```python
from build123d import *

# Parameters (mm, degrees)
SKETCH1_R           = 0.75
BOSS_EXTRUDE1_DEPTH = 2
SKETCH2_W           = 20.7
SKETCH2_H           = 2
SKETCH2_W_2         = 25.7
BOSS_EXTRUDE2_DEPTH = 4


with BuildPart() as part:
    # Sketch1 → Boss-Extrude1 (new body)
    # profile 1 of 3: a face of its own
    with BuildSketch(Plane(origin=(0, -22.368471217, 0), x_dir=(1, 0, 0), z_dir=(0, 1, 0))):
        Polygon((-7.325383597, 61.756641018), (1.674616403, 61.756641018), (1.674616403, 63.756641018), (-5.325383597, 63.756641018), (-5.325383597, 65.756641018), (-9.325383597, 65.756641018), (-9.325383597, 37.256641018), (-5.325383597, 37.256641018), (-5.325383597, 39.256641018), (1.674616403, 39.256641018), (1.674616403, 41.256641018), (-7.325383597, 41.256641018), align=None)
        with Locations(Location((-7.325383597, 63.756641018, 0), (0, 0, 270))):
            Circle(SKETCH1_R, mode=Mode.SUBTRACT)
        with Locations(Location((-7.325383597, 39.256641018, 0), (0, 0, 270))):
            Circle(SKETCH1_R, mode=Mode.SUBTRACT)
    # profile 2 of 3: a face of its own
    with BuildSketch(Plane(origin=(0, -22.368471217, 0), x_dir=(1, 0, 0), z_dir=(0, 1, 0))):
        Polygon((1.674616403, 39.256641018), (22.974616403, 39.256641018), (22.974616403, 41.256641018), (31.974616403, 41.256641018), (31.974616403, 61.756641018), (27.974616403, 61.756641018), (27.974616403, 63.756641018), (1.674616403, 63.756641018), (1.674616403, 61.756641018), (-7.325383597, 61.756641018), (-7.325383597, 41.256641018), (1.674616403, 41.256641018), align=None)
    # profile 3 of 3: a face of its own
    with BuildSketch(Plane(origin=(0, -22.368471217, 0), x_dir=(1, 0, 0), z_dir=(0, 1, 0))):
        Polygon((29.974616403, 65.756641018), (29.974616403, 63.756641018), (27.974616403, 63.756641018), (27.974616403, 61.756641018), (31.974616403, 61.756641018), (31.974616403, 41.256641018), (22.974616403, 41.256641018), (22.974616403, 39.256641018), (29.974616403, 39.256641018), (29.974616403, 37.256641018), (33.974616403, 37.256641018), (33.974616403, 65.756641018), align=None)
        with Locations(Location((31.974616403, 39.256641018, 0), (0, 0, 270))):
            Circle(SKETCH1_R, mode=Mode.SUBTRACT)
        with Locations(Location((31.974616403, 63.756641018, 0), (0, 0, 270))):
            Circle(SKETCH1_R, mode=Mode.SUBTRACT)
    extrude(amount=BOSS_EXTRUDE1_DEPTH)

    # Sketch2 → Boss-Extrude2 (add)
    with BuildSketch(Plane.XZ.offset(22.368471217)):
        with Locations((12.324616403, -40.256641018)):
            Rectangle(SKETCH2_W, SKETCH2_H)
        with Locations((14.824616403, -62.756641018)):
            Rectangle(SKETCH2_W_2, SKETCH2_H)
    extrude(amount=BOSS_EXTRUDE2_DEPTH)


solid = part.part
```
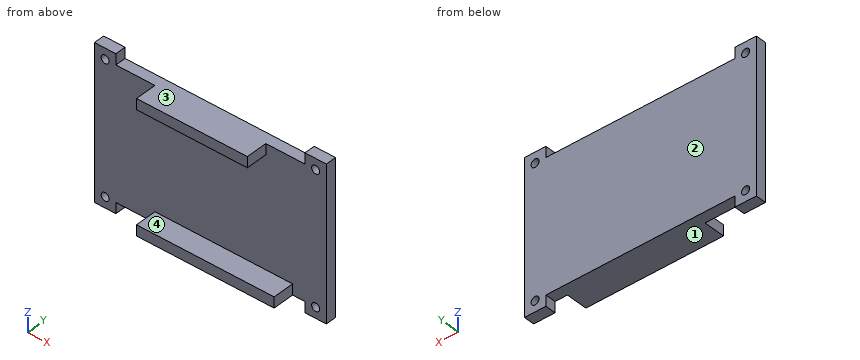
Input: part model. Units: mm. Frame: model coordinates. Face numbers are marked on the shaded views. A direction names the side the tool comes from. Give positions to 0.01 mm unless a question says otherwise; leave off trailing zeros. Loops run counter-clockwise (first coordinate to the right, second up) from the corner with the lowest first, then second, coordinate; pieces in that order, holes last.
1) Line query: L1, parallel to Z at x = 13, y = -24.05; L2, parallel to Y at x = 9, z = -47.75; L3, parallel to X at y = -22.75, z = -63. Output: solid intervals per line, ascending.
A:
L1: z = -63.76 to -61.76, -41.26 to -39.26
L2: y = -22.37 to -20.37
L3: x = 1.97 to 27.67
2) Section query B-B on x = 21.5. Return the cut outline in (y, z).
A:
outline: (-26.37, -63.76) - (-20.37, -63.76) - (-20.37, -39.26) - (-26.37, -39.26) - (-26.37, -41.26) - (-22.37, -41.26) - (-22.37, -61.76) - (-26.37, -61.76) - close
3) Contact query for flat-ended pins moving along their axis: pin 1 (2 mm diameter, centred on y = -24.5, z = -62.5, fed in from -X); pin 2 (3 mm diameter, centred on x = 14.5, y = -22, fed in from +Z); pin 3 (1.6 mm diameter, centred on y = -25, z = -40, fed in from +X). Output: stop coordinate, or through.
A:
pin 1: stops at x = 1.97
pin 2: stops at z = -39.26
pin 3: stops at x = 22.67
4) Section query D-D on x = -4. Return the cut outline in (y, z), and give its area (3 significant figures).
A:
outline: (-22.37, -63.76) - (-20.37, -63.76) - (-20.37, -39.26) - (-22.37, -39.26) - close
area: 49.0 mm2
5) Mould query, pull axis X, two halves, no side actions, for the marked faces 3 and 4. Classes: released by +X, released by -X, zero draft, split by the parting line, or undercut.
A:
face 3: undercut
face 4: zero draft
6) Reachability of the marked faces 1 and 2 from +Z, -Z, +X, -X, +Y, -Y: full face, straight path, thin tool, end or side. Return the list, or none.
A:
face 1: -Z, +Y, -Y
face 2: +Z, -Z, +X, -X, +Y
7) Section query A-A on y = -23.4. Return the cut outline in (x, z).
A:
outline: (1.97, -63.76) - (27.67, -63.76) - (27.67, -61.76) - (1.97, -61.76) - close; (1.97, -41.26) - (22.67, -41.26) - (22.67, -39.26) - (1.97, -39.26) - close
8) Section query C-C on z = -47.5. Return the cut outline in (x, y).
A:
outline: (-9.33, -22.37) - (33.97, -22.37) - (33.97, -20.37) - (-9.33, -20.37) - close
